CAD build for the part. Positions are in the model's coordinates, mm. Face numbers are marked on the shaded views. A direction names the side the tool comes from. Round coordinates to 2 decimals unless told otherwise and drop trailing zeros. Order: outer loops, then holes, each group sorted by start corner. A loop starts at its lowest first (then second) coordinate and runs counter-clockwise, first axis right, second up. Notation, with made-up numbers: M 81,-39 L 116,-39 A6 ccw 116,-29 Z; hole C 75,37.5 d9. An arc over 180 degrees is marked long. Answer as a JSON object with one key per item and string values.
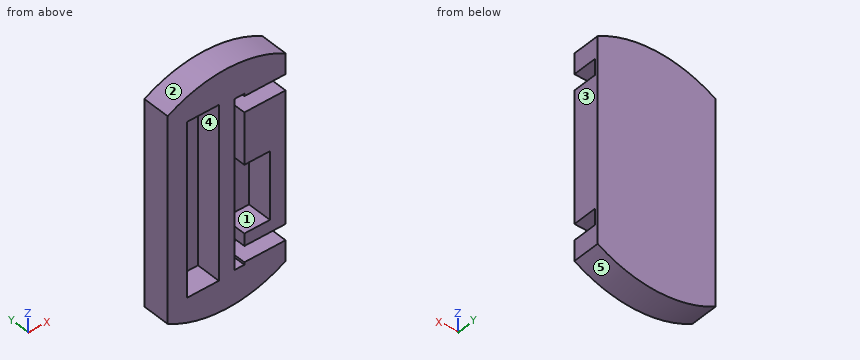
```python
from build123d import *

# Parameters (mm, degrees)
F0_R     = 38.1
F1_DEPTH = 8.89
F2_W     = 10.31875
F2_H     = 55.88
F3_DEPTH = 7.9375
F5_DEPTH = 7.9375
F6_W     = 39.77474
F6_H     = 108.857153
F7_DEPTH = 25.4


with BuildPart() as f1:
    # F0 (on Front) → F1 (new body)
    with BuildSketch(Plane.XZ):
        Circle(F0_R)
    extrude(amount=F1_DEPTH)

    # F2 (on face) → F3 (cut)
    with BuildSketch(Plane.XZ.offset(8.89)):
        with Locations((-7.699375, 0)):
            Rectangle(F2_W, F2_H)
    extrude(amount=-F3_DEPTH, mode=Mode.SUBTRACT)

    # F4 (on face) → F5 (cut)
    with BuildSketch(Plane.XZ.offset(8.89)):
        with BuildLine():
            Line((5.715, 27.178), (2.54, 27.178))
            Line((2.54, 27.178), (2.54, -27.178))
            Line((2.54, -27.178), (5.715, -27.178))
            Line((5.715, -27.178), (5.715, -26.38425))
            Line((5.715, -26.38425), (12.12081, -26.38425))
            Line((12.12081, -26.38425), (27.486021, -26.38425))
            ThreePointArc((27.486021, -26.38425), (29.675547, -23.895018), (31.640396, -21.224875))
            Line((31.640396, -21.224875), (13.97, -21.224875))
            Line((13.97, -21.224875), (12.12081, -21.224875))
            Line((12.12081, -21.224875), (5.715, -21.224875))
            Line((5.715, -21.224875), (5.715, -17.256125))
            Line((5.715, -17.256125), (13.97, -17.256125))
            Line((13.97, -17.256125), (13.97, 4.572))
            Line((13.97, 4.572), (5.715, 4.572))
            Line((5.715, 4.572), (5.715, 21.224875))
            Line((5.715, 21.224875), (12.12081, 21.224875))
            Line((12.12081, 21.224875), (13.97, 21.224875))
            Line((13.97, 21.224875), (31.640396, 21.224875))
            ThreePointArc((31.640396, 21.224875), (29.675547, 23.895018), (27.486021, 26.38425))
            Line((27.486021, 26.38425), (12.12081, 26.38425))
            Line((12.12081, 26.38425), (5.715, 26.38425))
            Line((5.715, 26.38425), (5.715, 27.178))
        make_face()
    extrude(amount=-F5_DEPTH, mode=Mode.SUBTRACT)

    # F6 (on face) → F7 (cut)
    with BuildSketch(Plane.XZ.offset(8.89)):
        with Locations((38.93737, -0.989815)):
            Rectangle(F6_W, F6_H)
        with Locations((-38.93737, -0.989815)):
            Rectangle(F6_W, F6_H)
    extrude(amount=-F7_DEPTH, mode=Mode.SUBTRACT)


solid = f1.part
```
Item 1: Saw through at B-B on z = 22. List the corners of the cut face in (x, y).
Worked answers:
{"outline": "M -19.05,-8.89 L -12.86,-8.89 L -12.86,-0.95 L -2.54,-0.95 L -2.54,-8.89 L 2.54,-8.89 L 2.54,-0.95 L 19.05,-0.95 L 19.05,0 L -19.05,0 Z"}
Item 2: Saw through at A-A on y = -2. List the corners of the cut face in (x, z) (3 decimals).
Worked answers:
{"outline": "M -19.05,-32.996 A38.1 ccw 19.05,-32.996 L 19.05,-26.384 L 5.715,-26.384 L 5.715,-27.178 L 2.54,-27.178 L 2.54,27.178 L 5.715,27.178 L 5.715,26.384 L 19.05,26.384 L 19.05,32.996 A38.1 ccw -19.05,32.996 Z; M 5.715,-21.225 L 19.05,-21.225 L 19.05,21.225 L 5.715,21.225 L 5.715,4.572 L 13.97,4.572 L 13.97,-17.256 L 5.715,-17.256 Z; hole M -12.859,-27.94 L -2.54,-27.94 L -2.54,27.94 L -12.859,27.94 Z"}
Item 3: Drop flat-ended pins along their axis: pin 1 Ø2.5 at (x, y) = (3.5, -3.5) entering from -Z; pin 2 Ø1.5 at (x, y) = (-8, -1.5) entering from -Z; pin 3 Ø4 at (x, y) = (10, -5.5) entering from +Z. Give the stop position or say it passes through.
Worked answers:
{"pin 1": "stops at z = -38.03", "pin 2": "stops at z = -37.4", "pin 3": "stops at z = 37.25"}
Item 4: Wall check: line 1 along X through (y, z) = (-8, -9.5); line 2 along X through (y, z) = (-2, 27) (3 decimals); line 3 along X through (y, z) = (-2.75, -26). Give the ranges that are in metal, low to high. Write a range as [from, to].
Worked answers:
{"line 1": "x = [-19.05, -12.86], [-2.54, 2.54], [13.97, 19.05]", "line 2": "x = [-19.05, -12.859], [-2.54, 2.54], [5.715, 19.05]", "line 3": "x = [-19.05, -12.86], [-2.54, 2.54]"}
Item 5: Saw through at C-C on x = 15.5. List the corners of the cut face in (y, z), and give its area (3 significant figures).
Worked answers:
{"outline": "M -8.89,-34.8 L 0,-34.8 L 0,34.8 L -8.89,34.8 L -8.89,26.38 L -0.95,26.38 L -0.95,21.22 L -8.89,21.22 L -8.89,-21.22 L -0.95,-21.22 L -0.95,-26.38 L -8.89,-26.38 Z", "area": "537 mm2"}
Item 6: Two-plate mould, pull along X, no slides. Class the marked faces 1, 2 and 3: released by +X, released by -X, zero draft, split by the parting line, or undercut.
Worked answers:
{"face 1": "undercut", "face 2": "split by the parting line", "face 3": "released by +X"}
Item 7: 3-axis set-ups, long thin cutter, end or side, ignore diameter. For the marked faces 4 and 5: which of +Z, -Z, +X, -X, +Y, -Y reach the whole face in a straight line?
Worked answers:
{"face 4": "-Y", "face 5": "-Z, +Y, -Y"}
